Model file for the job. Use its own axes, mm. A direction names the side the tool comes from. Round coordinates to 2 decimals unless told otherwise and drop trailing zeros. Order: outer loops, then holes, each group sorted by start corner. A loop starts at its lowest first (then second) coordinate and runs counter-clockwise, first axis right, second up. Notation, with made-up numbers: (34.5, 5.5) - (41.5, 5.5) arc R25 cw to (41.5, 26.5) - close; hole circle Ø2 at (53, 57). An arc over 180 degrees is marked (long way). Use one line per item in the form item = value.
from build123d import *

# Parameters (mm, degrees)
SKETCH1_W           = 10
SKETCH1_H           = 10
BOSS_EXTRUDE1_DEPTH = 65
CUT_EXTRUDE1_DEPTH  = 5


with BuildPart() as part:
    # Sketch1 → Boss-Extrude1 (new body)
    with BuildSketch(Plane.XY):
        with Locations((-11.829268293, -0.975609756)):
            Rectangle(SKETCH1_W, SKETCH1_H)
    extrude(amount=BOSS_EXTRUDE1_DEPTH)

    # Sketch2 → Cut-Extrude1 (cut)
    with BuildSketch(Plane.XY.offset(65)):
        Polygon((-9.329268293, 1.524390244), (-11.829268293, 4.024390244), (-16.829268293, 4.024390244), (-16.829268293, -3.475609756), (-9.329268293, -3.475609756), align=None)
        Polygon((-9.329268293, 4.024390244), (-11.829268293, 4.024390244), (-9.329268293, 1.524390244), align=None)
    extrude(amount=-CUT_EXTRUDE1_DEPTH, mode=Mode.SUBTRACT)


solid = part.part
(1) Probe probe 1 along Z at (x, y) = (-10.5, 3.5); probe 2 along Y at (x, z) = (-13.75, 61). List the from-to ranges inside material, lowest first. Write a range as [from, to].
Report:
probe_1 = [0, 60]
probe_2 = [-5.98, -3.48]
(2) Slice it at A-A on y = -1.5. Give the cut face in (x, z), then the cut area to 4 significant figures.
Report:
outline = (-16.83, 0) - (-6.83, 0) - (-6.83, 65) - (-9.33, 65) - (-9.33, 60) - (-16.83, 60) - close
area = 612.5 mm2
(3) Pin check, flat tips, straight feed: pin 1 (1.5 mm diameter, centred on y = -1, z = 62.5, fed in from -X); pin 2 (5 mm diameter, centred on x = -12.5, y = 2.5, fed in from +Z). Stop position of each tip, or through.
Report:
pin_1 = -9.33
pin_2 = 60
(4) Tool access for faces 1 (the face through (-12, -5.976, 32)), 2 (the face through (-13, -3.476, 63)): list every direction of +Z, -Z, +X, -X, +Y, -Y with a clear straight run to the whole face (end or side of a thin tool).
Report:
face_1 = +Z, -Z, +X, -X, -Y
face_2 = +Z, -X, +Y
(5) Slice it at B-B on z = 61. Give the cut face in (x, y), then the cut area to 4 significant figures.
Report:
outline = (-16.83, -5.98) - (-6.83, -5.98) - (-6.83, 4.02) - (-9.33, 4.02) - (-9.33, -3.48) - (-16.83, -3.48) - close
area = 43.75 mm2
